Source: CAD feature listing. Evaluate the final solid. Frame: model axes, mm. Give positions to 0.01 mm unless a question says otherwise; leave off trailing zeros. Write each loop counter-clockwise with the first axis right and the second up, starting at its lowest first coordinate (ties: lowest second). Pieces come first, ordered by that corner, then holes.
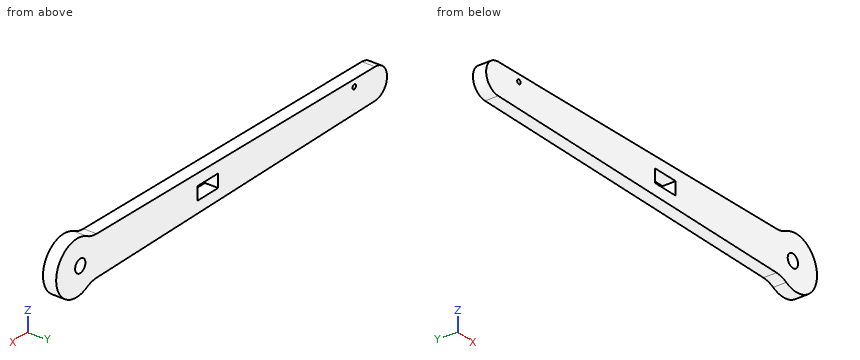
```python
from build123d import *

# Parameters (mm, degrees)
CROQUIS1_R                 = 0.5
CROQUIS1_R_2               = 1.5
CROQUIS1_W                 = 6
CROQUIS1_H                 = 3
SALIENTE_EXTRUIR1_DEPTH    = 3
S_LIDO_MOVER_COPIAR1_ANGLE = 90


with BuildPart() as part:
    # Croquis1 → Saliente-Extruir1 (new body)
    with BuildSketch(Plane.XY):
        with BuildLine():
            Line((41811.264601562, -420.544949858), (41892.031527809, -419.541772165))
            ThreePointArc((41892.031527809, -419.541772165), (41893.493281322, -419.343004838), (41894.86235293, -418.793573574))
            ThreePointArc((41894.86235293, -418.793573574), (41903.764601562, -424.044949858), (41894.86235293, -429.296326142))
            ThreePointArc((41894.86235293, -429.296326142), (41893.493281322, -428.746894878), (41892.031527809, -428.548127552))
            Line((41892.031527809, -428.548127552), (41811.264601555, -427.544949858))
            ThreePointArc((41811.264601555, -427.544949858), (41807.764601562, -424.044949855), (41811.264601562, -420.544949858))
        make_face()
        with Locations((41817.264601562, -426.044949857)):
            Circle(CROQUIS1_R, mode=Mode.SUBTRACT)
        with Locations((41896.764601562, -424.044949858)):
            Circle(CROQUIS1_R_2, mode=Mode.SUBTRACT)
        with Locations((41859.764601562, -424.044949858)):
            Rectangle(CROQUIS1_W, CROQUIS1_H, mode=Mode.SUBTRACT)
    extrude(amount=SALIENTE_EXTRUIR1_DEPTH)


with BuildPart() as part_1:
    # Sólido-Mover/Copiar1: moved
    add(part.part.rotate(Axis((0, -424.044949858, 1.5), (-1, 0, 0)), S_LIDO_MOVER_COPIAR1_ANGLE))


solid = part_1.part
```
1. Section query B-B (z = 1.5). Return loops of the section in (x, y).
2. Section query C-C (x = 41828.5). Return loops of the section in (y, z), plus the area to 3 significant figures.
3. Pin query (flat end, axial travel): P1, Ø5, axis at x = 41896.76, z = 1.5, coming from the -Y side; P2, Ø1.5, axis at x = 41859, y = -424.5, coming from the -Z side; P3, Ø1, axis at x = 41822, y = -424, coming from the -Z side. Return the tip coordinate at first contact, or that it passes through.
4. Section query D-D (x = 41887). Return loops of the section in (y, z).
5. Section query A-A (y = -424.3). Return loops of the section in (x, z).
6. Line query: probe 1 along X at (y, z) = (-424, 1.5); probe 2 along X at (y, z) = (-424.15, 2.5); probe 3 along Z at (x, y) = (41859, -422.9). Output: solid intervals per line, ascending.
The answers:
1. outline: (41807.76, -425.54) - (41856.76, -425.54) - (41856.76, -422.54) - (41807.76, -422.54) - close; (41862.76, -425.54) - (41895.26, -425.54) - (41895.26, -422.54) - (41862.76, -422.54) - close; (41898.26, -425.54) - (41903.76, -425.54) - (41903.76, -422.54) - (41898.26, -422.54) - close
2. outline: (-425.54, -2.21) - (-422.54, -2.21) - (-422.54, 5.21) - (-425.54, 5.21) - close
2. area: 22.3 mm2
3. P1: stops at y = -425.54
3. P2: stops at z = -2.6
3. P3: stops at z = -2.14
4. outline: (-425.54, -2.94) - (-422.54, -2.94) - (-422.54, 5.94) - (-425.54, 5.94) - close
5. outline: (41811.26, -2) - (41892.03, -3) arc R6 cw to (41894.86, -3.75) arc R6 ccw (long way) to (41894.86, 6.75) arc R6 cw to (41892.03, 6) - (41811.26, 5) arc R3.5 ccw to start; hole circle Ø1 at (41817.26, 3.5); hole (41856.76, 0) - (41862.76, 0) - (41862.76, 3) - (41856.76, 3) - close; hole circle Ø3 at (41896.76, 1.5)
6. probe 1: x = 41807.76 to 41856.76, 41862.76 to 41895.26, 41898.26 to 41903.76
6. probe 2: x = 41807.91 to 41856.76, 41862.76 to 41895.65, 41897.88 to 41903.68
6. probe 3: z = -2.59 to 0, 3 to 5.59
